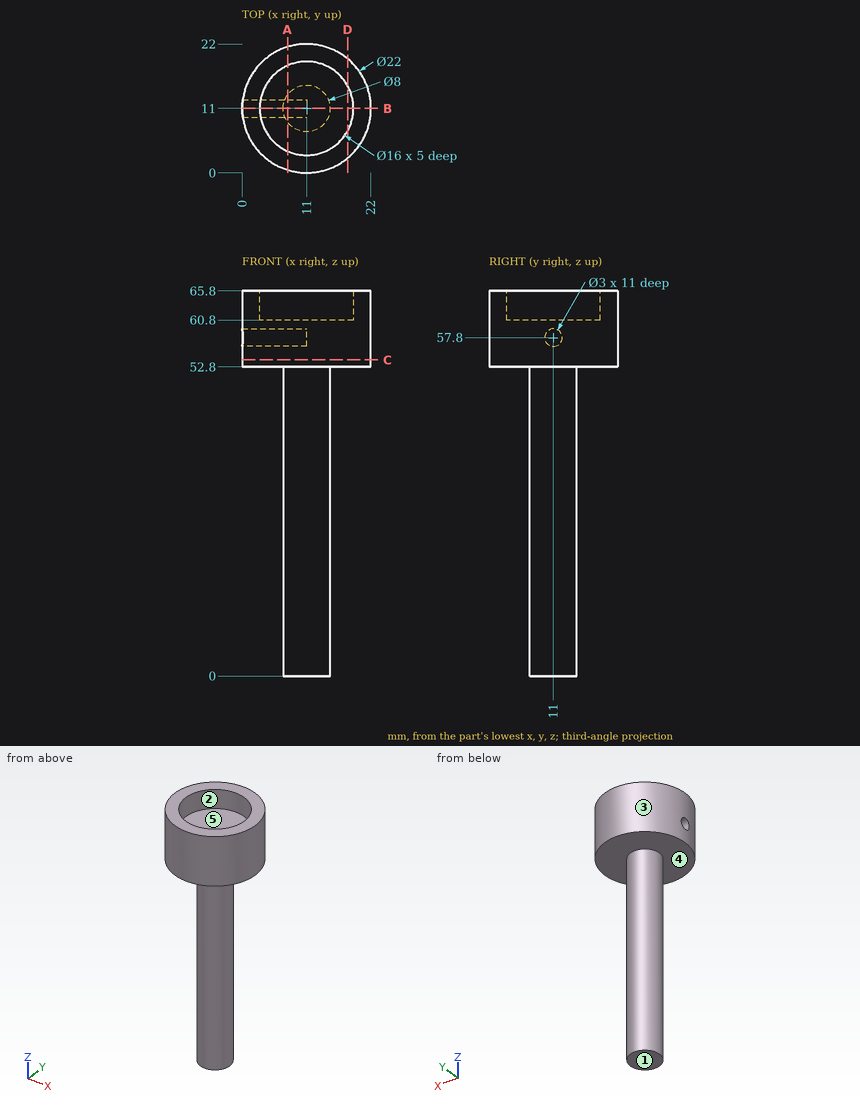
Geometry: see drawing. Coordinates: mm, zero at the bounding-box minimum. A direction names the side the tool comes from. Round coordinates to 2 decimals unless told otherwise and drop trailing zeros. Loops run counter-clockwise (first coordinate to the right, second up) from the corner with the lowest first, then second, coordinate; pieces in that order, holes last. Notation, with made-up numbers: (24, 53.25) - (43, 53.25) arc R18 ccw to (43, 69.25) - close; hole circle Ø2 at (-8.75, 62.5). An arc over 180 degrees is marked (long way). One line per item, written item: value. Start each with the question number.
(1) Section A-A, the plane x = 7.75. Return loops of the section in (y, z), plus the area to 3 significant figures.
(2) Section D-D, the plane x = 18. Return loops of the section in (y, z).
(3) Access query for the marked faces 4 and 5. Directions: +Z, -Z, +X, -X, +Y, -Y. A direction counts if a zero-diameter tool reaches every point of the face in a straight line with its end or side. Return the directions, or none.
(4) Draft query along Y for the marked faces 1, 2 and 3. Return one class per face: +Y half, -Y half, draft (parallel to the pull), parting line (faces both ways), or undercut.
(5) Ray query, line 1 (Y direction, x = 11, z = 63.2); line 2 (Z direction, x = 5, y = 15.5); line 3 (Z direction, x = 15.5, y = 4). Return the intervals inside material, ascending. Write a range as [from, to].
(6) Section C-C, the plane z = 54. Return loops of the section in (x, y).
(7) Contact query for flat-ended pins moving along their axis: P1, Ø3, axis at y = 12.5, z = 53, coming from the +X side; P2, Ø1.5, axis at y = 11, z = 58, coming from the -X side; P3, Ø10, axis at y = 14, z = 27.5, coming from the -X side; P4, Ø2, axis at x = 13.5, z = 25, coming from the +Y side. Output: stop coordinate, or through.
(8) Section B-B, the plane y = 11. Return loops of the section in (x, z).
Results below:
1. outline: (0.49, 52.8) - (8.67, 52.8) - (8.67, 0) - (13.33, 0) - (13.33, 52.8) - (21.51, 52.8) - (21.51, 65.8) - (18.31, 65.8) - (18.31, 60.8) - (3.69, 60.8) - (3.69, 65.8) - (0.49, 65.8) - close; hole circle Ø3 at (11, 57.8)
1. area: 439 mm^2
2. outline: (2.51, 52.8) - (19.49, 52.8) - (19.49, 65.8) - (14.87, 65.8) - (14.87, 60.8) - (7.13, 60.8) - (7.13, 65.8) - (2.51, 65.8) - close
3. face 4: -Z
3. face 5: +Z
4. face 1: draft
4. face 2: undercut
4. face 3: parting line
5. line 1: [0, 3], [19, 22]
5. line 2: [52.8, 60.8]
5. line 3: [52.8, 65.8]
6. outline: circle Ø22 at (11, 11)
7. P1: x = 22
7. P2: x = 11
7. P3: x = 7
7. P4: y = 14.71
8. outline: (0, 52.8) - (7, 52.8) - (7, 0) - (15, 0) - (15, 52.8) - (22, 52.8) - (22, 65.8) - (19, 65.8) - (19, 60.8) - (3, 60.8) - (3, 65.8) - (0, 65.8) - (0, 59.3) - (11, 59.3) - (11, 56.3) - (0, 56.3) - close
